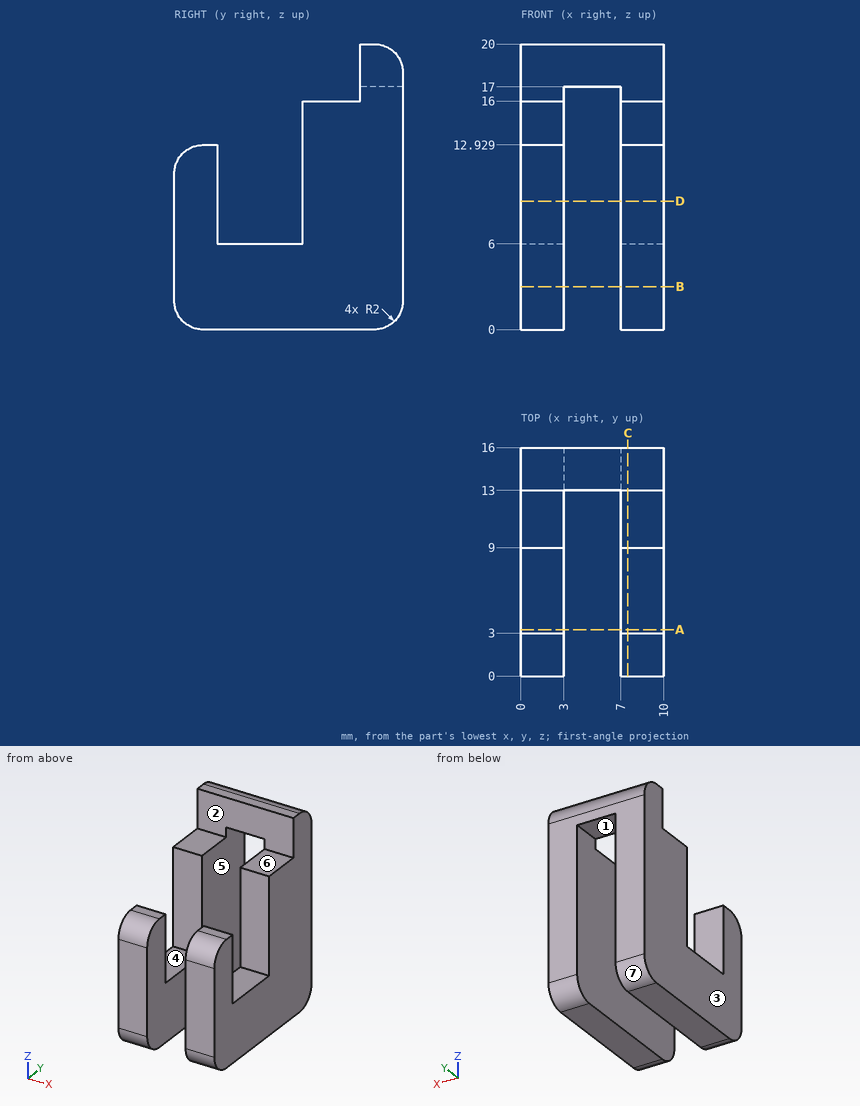
Geometry check sheet. Reference: drawing and pictorial views, mm from the part's lowest x, y, z. A direction names the side the tool comes from. Give positions to 0.01 mm unless a question says otherwise; leave off trailing zeros. Order: outer loops, then holes, each group sorted by start corner. A loop starts at its lowest first (then second) coordinate and runs counter-clockwise, first axis right, second up. Notation, with made-up numbers: M -23.75,11.25 L 23.25,11.25 A18 ccw 23.25,24.25 Z; hole C 24,68 d6. An arc over 180 degrees is marked long. Return JSON: item names as keys, results as strings. Group by question number.
1) Section check C-C on x = 7.5. Record the cut outline in (y, z).
2) Go/stop test with flat-tipped pins: pin 1 Ø0.5 at (x, y) = (1.5, 2.5) entering from +Z; pin 2 Ø1.5 at (y, z) = (12.5, 10) entering from -X; pin 3 Ø4.5 at (x, z) = (5, 19) entering from -Y; pin 4 Ø3.5 at (x, y) = (8.5, 10.5) entering from +Z. Record where each tip stops, or that it passes through.
3) Section check A-A on y = 3.25. Record the cut outline in (x, z), and give its area (3 significant figures).
4) Section check D-D on z = 9. Record the cut outline in (x, y).
5) Section check B-B on z = 3. Record the cut outline in (x, y).
6) Access from +Z, -Z, +X, -X, +Y, -Y to the whole of each face (thin tool, end or side, straight path). Record for the marked faces 4, 5, 6 and 7.
7) Mould release check, pull along X, two halves, no side actions. Record for the marked faces 1, 2 and 3: pulls with the +X half, pulls with the -X half, needs draft (parallel to the pull), parting line crosses it, or undercut.
8) Scan lines: line 1 (X direction, y = 13.25, z = 6.25); line 2 (Y direction, x = 0.5, z = 9.5); line 3 (Z direction, x = 7.5, y = 7). Record each from-to range of solid material in increasing order.
Answer block:
{
 "1": {"outline": "M 0,2 A2 ccw 2,0 L 14,0 A2 ccw 16,2 L 16,18 A2 ccw 14,20 L 13,20 L 13,16 L 9,16 L 9,6 L 3,6 L 3,12.93 L 2,12.93 A2 ccw 0,10.93 Z"},
 "2": {"pin 1": "stops at z = 12.93", "pin 2": "stops at x = 0", "pin 3": "stops at y = 13", "pin 4": "stops at z = 16"},
 "3": {"outline": "M 0,0 L 3,0 L 3,6 L 0,6 Z; M 7,0 L 10,0 L 10,6 L 7,6 Z", "area": "36.0 mm^2"},
 "4": {"outline": "M 0,0 L 3,0 L 3,3 L 0,3 Z; M 0,9 L 3,9 L 3,16 L 0,16 Z; M 7,0 L 10,0 L 10,3 L 7,3 Z; M 7,9 L 10,9 L 10,16 L 7,16 Z"},
 "5": {"outline": "M 0,0 L 3,0 L 3,16 L 0,16 Z; M 7,0 L 10,0 L 10,16 L 7,16 Z"},
 "6": {"face 4": "+Z, +X, -X", "face 5": "-Z, +Y, -Y", "face 6": "+Z, +X, -X, -Y", "face 7": "-Z, +X, -X, +Y"},
 "7": {"face 1": "undercut", "face 2": "needs draft", "face 3": "pulls with the -X half"},
 "8": {"line 1": "x = 0 to 3, 7 to 10", "line 2": "y = 0 to 3, 9 to 16", "line 3": "z = 0 to 6"}
}
